from build123d import *

# Parameters (mm, degrees)
BASE_FLANGE1_DEPTH = 6.35
SKETCH8_R          = 3.4
CUT_EXTRUDE1_DEPTH = 183.851914127
SKETCH9_R          = 18.5
CUT_EXTRUDE2_DEPTH = 183.851914127
SKETCH11_R         = 1.2
CUT_EXTRUDE4_DEPTH = 183.851914127


# Sheet-metal steps are written as plain solids
with BuildPart() as part:
    # Sketch2 → Base-Flange1 (new body)
    with BuildSketch(Plane(origin=(0, 0, 0), x_dir=(1, 0, 0), z_dir=(0, 1, 0))):
        with BuildLine():
            Line((0, 0), (50.76093065, 0))
            Line((50.76093065, 0), (107.880465325, 57.119534675))
            ThreePointArc((107.880465325, 57.119534675), (111.537953618, 118.761570635), (50.76093065, 129.682710556))
            Line((50.76093065, 129.682710556), (0, 90))
            Line((0, 90), (0, 0))
        make_face()
    extrude(amount=-BASE_FLANGE1_DEPTH)

    # Sketch8 → Cut-Extrude1 (cut, through all)
    with BuildSketch(Plane(origin=(0, 0, 0), x_dir=(1, 0, 0), z_dir=(0, 1, 0))):
        with Locations(Location((12.5, 79, 0), (0, 0, 270))):
            Circle(SKETCH8_R)
        with Locations(Location((12.5, 11, 0), (0, 0, 90))):
            Circle(SKETCH8_R)
    extrude(amount=-CUT_EXTRUDE1_DEPTH, mode=Mode.SUBTRACT)

    # Sketch9 → Cut-Extrude2 (cut, through all)
    with BuildSketch(Plane(origin=(0, 0, 0), x_dir=(1, 0, 0), z_dir=(0, 1, 0))):
        with Locations(Location((75, 90, 0), (0, 0, 270))):
            Circle(SKETCH9_R)
    extrude(amount=-CUT_EXTRUDE2_DEPTH, mode=Mode.SUBTRACT)

    # Sketch11 → Cut-Extrude4 (cut, through all)
    with BuildSketch(Plane(origin=(0, 0, 0), x_dir=(1, 0, 0), z_dir=(0, 1, 0))):
        with Locations(Location((17.5, 25, 0), (0, 0, 270))):
            Circle(SKETCH11_R)
        with Locations(Location((17.5, 34.5, 0), (0, 0, 270))):
            Circle(SKETCH11_R)
    extrude(amount=-CUT_EXTRUDE4_DEPTH, mode=Mode.SUBTRACT)


solid = part.part
Check sheet for the modelled part. Datum: model origin and axes. Units: mm. Give positions to 0.01 mm unless a question says otherwise; leave off trailing zeros. Loops run counter-clockwise (first coordinate to the right, second up) from the corner with the lowest first, then second, coordinate; pieces in that order, holes last. Notation, with made-up numbers: M 45,80 L 78,80 A24 cw 78,104 Z; hole C 20,7.25 d6. An arc over 180 degrees is marked long. Return JSON: item names as keys, results as strings. Group by question number.
1. Cross-section at D-D on x = 12.5. Record the boundary of the cut face in (y, z), plus the area to 3 significant figures.
2. Thickness scan on L1, parallel to X at y = -1.5, z = -90; L2, parallel to X at y = -4.75, z = -10; L3, parallel to Z at x = 66.5, y = -4. Record the ranges inside material, lowest first.
3. Go/stop test with flat-tipped pins: pin 1 (2 mm diameter, centred on x = 96, y = -5, fed in from -Z); pin 2 (1 mm diameter, centred on y = -1.5, z = -53.5, fed in from +X). Record where each tip stops, or that it passes through.
4. Cross-section at A-A on y = -2.75. Record the boundary of the cut face in (x, z), plus the area to 3 significant figures.
5. Cross-section at C-C on x = 77.5. Record the boundary of the cut face in (y, z).
6. Cross-section at B-B on z = -79. Record the boundary of the cut face in (x, y).
7. Mould release check, pull along Z, two halves, no side actions. Record for faces 1 (the flat face through (0, -3, -46)), 2 (the flat face through (78.92, -3.13, -28.16)), 3 (the cylindrical face through (10.431, -3.131, -81.698)): released by +Z, released by -Z, zero draft, split by the parting line, or undercut.
Return value:
{
 "1": {"outline": "M -6.35,-99.77 L 0,-99.77 L 0,-82.4 L -6.35,-82.4 Z; M -6.35,-75.6 L 0,-75.6 L 0,-14.4 L -6.35,-14.4 Z; M -6.35,-7.6 L 0,-7.6 L 0,0 L -6.35,0 Z", "area": "547 mm^2"},
 "2": {"L1": "0 to 56.5, 93.5 to 121.5", "L2": "0 to 9.25, 15.75 to 60.76", "L3": "-135.72 to -106.43, -73.57 to -15.74"},
 "3": {"pin 1": "z = -131.98", "pin 2": "x = 104.76"},
 "4": {"outline": "M 0,-90 L 50.76,-129.68 A46.5 ccw 107.88,-57.12 L 50.76,0 L 0,0 Z; hole C 12.5,-79 d6.8; hole C 12.5,-11 d6.8; hole C 17.5,-34.5 d2.4; hole C 17.5,-25 d2.4; hole C 75,-90 d37", "area": "11,000 mm^2"},
 "5": {"outline": "M -6.35,-136.43 L 0,-136.43 L 0,-108.33 L -6.35,-108.33 Z; M -6.35,-71.67 L 0,-71.67 L 0,-26.74 L -6.35,-26.74 Z"},
 "6": {"outline": "M 0,-6.35 L 9.1,-6.35 L 9.1,0 L 0,0 Z; M 15.9,-6.35 L 60.13,-6.35 L 60.13,0 L 15.9,0 Z; M 89.87,-6.35 L 120.18,-6.35 L 120.18,0 L 89.87,0 Z"},
 "7": {"face 1": "zero draft", "face 2": "released by +Z", "face 3": "undercut"}
}
